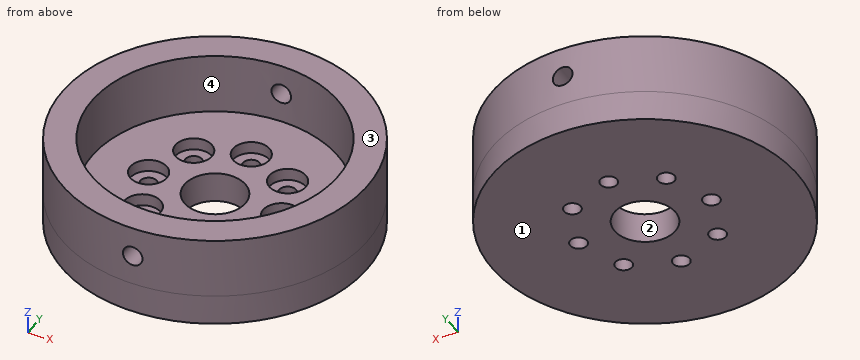
from build123d import *

# Parameters (mm, degrees)
SKETCH1_R               = 25
SKETCH1_R_2             = 20.15
BOSS_EXTRUDE1_DEPTH     = 10
BOSS_EXTRUDE2_START     = 5
SKETCH2_R               = 25
SKETCH2_R_2             = 1.375
SKETCH2_R_3             = 5
BOSS_EXTRUDE2_DEPTH     = 5
SKETCH3_R               = 3
CUT_EXTRUDE1_DEPTH      = 2
CUT_EXTRUDE2_DEPTH      = 38
CUT_EXTRUDE2_DEPTH_BACK = 33
SKETCH4_R               = 1.625


with BuildPart() as part:
    # Sketch1 → Boss-Extrude1 (new body)
    with BuildSketch(Plane.XY):
        Circle(SKETCH1_R)
        Circle(SKETCH1_R_2, mode=Mode.SUBTRACT)
    extrude(amount=BOSS_EXTRUDE1_DEPTH)

    # Sketch2 → Boss-Extrude2 (add)
    with BuildSketch(Plane(origin=(0, 0, 0), x_dir=(-1, 0, 0), z_dir=(0, 0, -1)).offset(BOSS_EXTRUDE2_START)):
        Circle(SKETCH2_R)
        with Locations((-11, 0)):
            Circle(SKETCH2_R_2, mode=Mode.SUBTRACT)
        with Locations((-7.778174593, 7.778174593)):
            Circle(SKETCH2_R_2, mode=Mode.SUBTRACT)
        with Locations((0, 11)):
            Circle(SKETCH2_R_2, mode=Mode.SUBTRACT)
        with Locations((7.778174593, 7.778174593)):
            Circle(SKETCH2_R_2, mode=Mode.SUBTRACT)
        with Locations((11, 0)):
            Circle(SKETCH2_R_2, mode=Mode.SUBTRACT)
        with Locations((7.778174593, -7.778174593)):
            Circle(SKETCH2_R_2, mode=Mode.SUBTRACT)
        with Locations((0, -11)):
            Circle(SKETCH2_R_2, mode=Mode.SUBTRACT)
        with Locations((-7.778174593, -7.778174593)):
            Circle(SKETCH2_R_2, mode=Mode.SUBTRACT)
        Circle(SKETCH2_R_3, mode=Mode.SUBTRACT)
    extrude(amount=-BOSS_EXTRUDE2_DEPTH)

    # Sketch3 → Cut-Extrude1 (cut)
    with BuildSketch(Plane.XY):
        with Locations((0, 11)):
            Circle(SKETCH3_R)
        with Locations((7.778174593, 7.778174593)):
            Circle(SKETCH3_R)
        with Locations((11, 0)):
            Circle(SKETCH3_R)
        with Locations((7.778174593, -7.778174593)):
            Circle(SKETCH3_R)
        with Locations((0, -11)):
            Circle(SKETCH3_R)
        with Locations((-7.778174593, -7.778174593)):
            Circle(SKETCH3_R)
        with Locations((-11, 0)):
            Circle(SKETCH3_R)
        with Locations((-7.778174593, 7.778174593)):
            Circle(SKETCH3_R)
    extrude(amount=-CUT_EXTRUDE1_DEPTH, mode=Mode.SUBTRACT)

    # Sketch4 → Cut-Extrude2 (cut, two sides: drawn at the far end of the back side and taken through both)
    with BuildSketch(Plane(origin=(0, 0, 0), x_dir=(1, 0, 0), z_dir=(0, 1, 0)).offset(-CUT_EXTRUDE2_DEPTH_BACK)):
        with Locations(Location((0, -5, 0), (0, 0, 90))):
            Circle(SKETCH4_R)
    extrude(amount=CUT_EXTRUDE2_DEPTH + CUT_EXTRUDE2_DEPTH_BACK, mode=Mode.SUBTRACT)


solid = part.part
Read the model definition and answer for the solid it produces. Units are mm, in the model's axes. Face numbers are marked on the shaded views. A direction names the side the tool comes from. Coordinates: 2 decimals unless noted, no trailing zeros. Loops run counter-clockwise (first coordinate to the right, second up) from the corner with the lowest first, then second, coordinate; pieces in that order, holes last. Notation, with made-up numbers: (-17, 89) -> (-13, 89) arc R11 cw to (-13, 105) -> close; hole circle Ø11 at (32, 53.25). An arc over 180 degrees is marked (long way). Write item = value, one per line. Start each with the question number.
1) The part is cut by section D-D, the plane x = -17. Determine the outline of the cut face in (y, z), plus the area to 3 significant figures.
2) Given P1, Ø6.5, axis at x = -7, y = 8, coming from the +Z side; P2, Ø6, axis at x = -11.5, z = -1, coming from the -Y side; P3, Ø5, axis at x = -7.78, y = -7.78, coming from the +Z side, each flat-ended and moving along its own axis, determine where each tip first touches the part or whether it passes through.
3) The part is cut by section B-B, the plane x = -7. Determine the outline of the cut face in (y, z), plus the area to 3 significant figures.
4) For the marked faces 3 and 4, determine the directions among +Z, -Z, +X, -X, +Y, -Y from which every point of the face is accessible in a straight line to the end or side of a thin tool.
5) The part is cut by section A-A, the plane y = 0. Determine the outline of the cut face in (x, z) (3 decimals), plus the area to 4 significant figures.
6) The mould has two halves that part along X. Classify the marked faces 1 and 2: pulls with the +X half, pulls with the -X half, needs draft (parallel to the pull), parting line crosses it, or undercut.
7) Find the intervals of material crossed by L1, parallel to Y at x = 0, z = -2.95 (3 decimals); L2, parallel to Y at x = 0, z = 2.5; L3, parallel to X at y = 0.5, z = 3.25 (3 decimals), in increasing order. Write a range as from..to.
8) The part is cut by section C-C, the plane z = 2.75. Determine the outline of the cut face in (x, y).
Result:
q1.outline = (-18.33, -5) -> (18.33, -5) -> (18.33, 10) -> (10.82, 10) -> (10.82, 0) -> (-10.82, 0) -> (-10.82, 10) -> (-18.33, 10) -> close
q1.area = 334 mm²
q2.P1 = 0
q2.P2 = -23.51
q2.P3 = -2
q3.outline = (-24, -5) -> (-8.91, -5) -> (-8.91, -2) -> (-10.68, -2) -> (-10.68, 0) -> (-18.9, 0) -> (-18.9, 10) -> (-24, 10) -> close; (-6.64, -5) -> (6.64, -5) -> (6.64, -2) -> (4.88, -2) -> (4.88, 0) -> (-4.88, 0) -> (-4.88, -2) -> (-6.64, -2) -> close; (8.91, -5) -> (24, -5) -> (24, 10) -> (18.9, 10) -> (18.9, 0) -> (10.68, 0) -> (10.68, -2) -> (8.91, -2) -> close
q3.area = 305 mm²
q4.face_3 = +Z, +X, -X, +Y, -Y
q4.face_4 = +Z
q5.outline = (-25, -5) -> (-12.375, -5) -> (-12.375, -2) -> (-14, -2) -> (-14, 0) -> (-20.15, 0) -> (-20.15, 10) -> (-25, 10) -> close; (-9.625, -5) -> (-5, -5) -> (-5, 0) -> (-8, 0) -> (-8, -2) -> (-9.625, -2) -> close; (5, -5) -> (9.625, -5) -> (9.625, -2) -> (8, -2) -> (8, 0) -> (5, 0) -> close; (12.375, -5) -> (25, -5) -> (25, 10) -> (20.15, 10) -> (20.15, 0) -> (14, 0) -> (14, -2) -> (12.375, -2) -> close
q5.area = 256.5 mm²
q6.face_1 = needs draft
q6.face_2 = undercut
q7.L1 = -25..-12.375, -9.625..-5, 5..9.625, 12.375..25
q7.L2 = -25..-20.15, 20.15..25
q7.L3 = -24.995..-20.144, 20.144..24.995
q8.outline = circle Ø50 at (0, 0); hole circle Ø40.3 at (0, 0)
